The model under review builds one solid part; all positions refer to its coordinate system, in mm. A direction names the side the tool comes from. Coordinates: 2 decimals unless noted, no trailing zeros. Write each loop counter-clockwise with the first axis right and the second up, starting at its lowest first coordinate (ties: lowest second). Pieces come first, ordered by that corner, then holes.
1) For line 1 (Y direction, x = 20, z = 15); line 2 (Y direction, x = 11.5, z = 53); line 3 (Z direction, x = 120, y = 79.5), list the stretches that pass through material, from the lowest coordinate up.
2) Add section C-C, the plane y = 129. State the section outline as (x, z) points.
3) Mouldability with a two-part tool opening along Y and no side actions: class faces 1 (the flat face through (69, 0, 9)), 2 (the cylindrical face through (86.94, 130.65, 6.25)), 3 (the cylindrical face through (40.4, 10.6, 49.1)) as released by +Y, released by -Y, zero draft, split by the parting line, or undercut.
4) For P1, Ø5.5, axis at y = 104.5, z = 8, coming from the -X side; P2, Ø2.5, axis at x = 44.5, y = 2, coming from the -Z side; P3, Ø16.5, axis at x = 101.5, y = 125.5, coming from the +Z side; P4, Ø9.5, axis at x = 35, z = 55, coming from the -Y side, all flat-tipped, find the tip position at first contact; note any pin that passes through.
5) Machinability: for faces 4 (the cylindrical face through (1.525, 63.66, 17.165)), 5 (the flat face through (83, 106, 24)), 6 (the flat face through (68.228, 106, 6)), which of the approach directions +Z, -Z, +X, -X, +Y, -Y give a long, thin tool a straight path to every point of the face, cutting with its end or side? Answer none if there is none.
6) Add section D-D, the plane x = 105. State the section outline as (y, z) points.
7) Add section A-A, the plane z = 55. State the section outline as (x, y) points, then the cut area to 3 significant figures.
8) Add section B-B, the plane x = 88. State the section outline as (y, z) points.
from build123d import *

# Parameters (mm, degrees)
BOSS_EXTRUDE1_DEPTH = 12
SKETCH1_3_R         = 20
SKETCH1_3_R_2       = 9
BOSS_EXTRUDE2_DEPTH = 24
SKETCH1_4_W         = 140
SKETCH1_4_H         = 18
BOSS_EXTRUDE3_DEPTH = 85
SKETCH2_R           = 27.5
SKETCH2_R_2         = 15
BOSS_EXTRUDE4_DEPTH = 18
SKETCH3_R           = 8
CUT_EXTRUDE1_DEPTH  = 208.560232222
SKETCH5_W           = 49
SKETCH5_H           = 3
CUT_EXTRUDE2_DEPTH  = 220.078182392


with BuildPart() as part:
    # Sketch1 → Boss-Extrude1 (new body)
    with BuildSketch(Plane.XY):
        with BuildLine():
            Line((140, 18), (123.22800697, 118))
            ThreePointArc((123.22800697, 118), (95.72800697, 90.5), (68.22800697, 118))
            Line((68.22800697, 118), (68.22800697, 101))
            ThreePointArc((68.22800697, 101), (60.9056765, 83.32233047), (43.22800697, 76))
            Line((43.22800697, 76), (20, 76))
            ThreePointArc((20, 76), (34.142135624, 70.142135624), (40, 56))
            ThreePointArc((40, 56), (20, 36), (0, 56))
            Line((0, 56), (0, 18))
            Line((0, 18), (140, 18))
        make_face()
    extrude(amount=BOSS_EXTRUDE1_DEPTH)

    # Sketch1_3 → Boss-Extrude2 (add)
    with BuildSketch(Plane.XY):
        with Locations(Location((20, 56, 0), (0, 0, 180))):
            Circle(SKETCH1_3_R)
        with Locations((20, 56)):
            Circle(SKETCH1_3_R_2, mode=Mode.SUBTRACT)
    extrude(amount=BOSS_EXTRUDE2_DEPTH)

    # Sketch1_4 → Boss-Extrude3 (add)
    with BuildSketch(Plane.XY):
        with Locations((70, 9)):
            Rectangle(SKETCH1_4_W, SKETCH1_4_H)
    extrude(amount=BOSS_EXTRUDE3_DEPTH)

    # Sketch2 → Boss-Extrude4 (add, symmetric)
    with BuildSketch(Plane(origin=(0, 0, 6), x_dir=(-1, 0, 0), z_dir=(0, 0, -1))):
        with Locations((-95, 118)):
            Circle(SKETCH2_R)
        with Locations((-95, 118)):
            Circle(SKETCH2_R_2, mode=Mode.SUBTRACT)
    extrude(amount=BOSS_EXTRUDE4_DEPTH, both=True)

    # Sketch3 → Cut-Extrude1 (cut, through all)
    with BuildSketch(Plane(origin=(0, 18, 0), x_dir=(1, 0, 0), z_dir=(0, 1, 0))):
        with Locations(Location((105, -55, 0), (0, 0, 270))):
            Circle(SKETCH3_R)
        with Locations(Location((35, -55, 0), (0, 0, 270))):
            Circle(SKETCH3_R)
    extrude(amount=-CUT_EXTRUDE1_DEPTH, mode=Mode.SUBTRACT)

    # Sketch5 → Cut-Extrude2 (cut, through all)
    with BuildSketch(Plane.ZY):
        with Locations((42.5, 1.5)):
            Rectangle(SKETCH5_W, SKETCH5_H)
    extrude(amount=-CUT_EXTRUDE2_DEPTH, mode=Mode.SUBTRACT)


solid = part.part
Geometry results:
1. line 1: y = 0 to 18, 36 to 47, 65 to 76
1. line 2: y = 3 to 18
1. line 3: z = 0 to 12
2. outline: (69.8, -12) - (84.8, -12) - (84.8, 24) - (69.8, 24) - close; (105.2, -12) - (120.2, -12) - (120.2, 24) - (105.2, 24) - close
3. face 1: released by -Y
3. face 2: undercut
3. face 3: zero draft
4. P1: stops at x = 68.23
4. P2: stops at z = 0
4. P3: stops at z = 24
4. P4: passes through
5. face 4: +Z
5. face 5: +Z, +X, -X, +Y
5. face 6: +Z, -Z, -X
6. outline: (0, 0) - (92.11, 0) - (92.11, 12) - (18, 12) - (18, 47) - (3, 47) - (3, 18) - (0, 18) - close; (0, 67) - (3, 67) - (3, 63) - (18, 63) - (18, 85) - (0, 85) - close; (92.38, -12) - (106.82, -12) - (106.82, 24) - (92.38, 24) - close; (129.18, -12) - (143.62, -12) - (143.62, 24) - (129.18, 24) - close
7. outline: (0, 3) - (27, 3) - (27, 18) - (0, 18) - close; (43, 3) - (97, 3) - (97, 18) - (43, 18) - close; (113, 3) - (140, 3) - (140, 18) - (113, 18) - close
7. area: 1,620 mm2
8. outline: (0, 0) - (91.41, 0) - (91.41, -12) - (104.73, -12) - (104.73, 24) - (91.41, 24) - (91.41, 12) - (18, 12) - (18, 85) - (0, 85) - (0, 67) - (3, 67) - (3, 18) - (0, 18) - close; (131.27, -12) - (144.59, -12) - (144.59, 24) - (131.27, 24) - close
